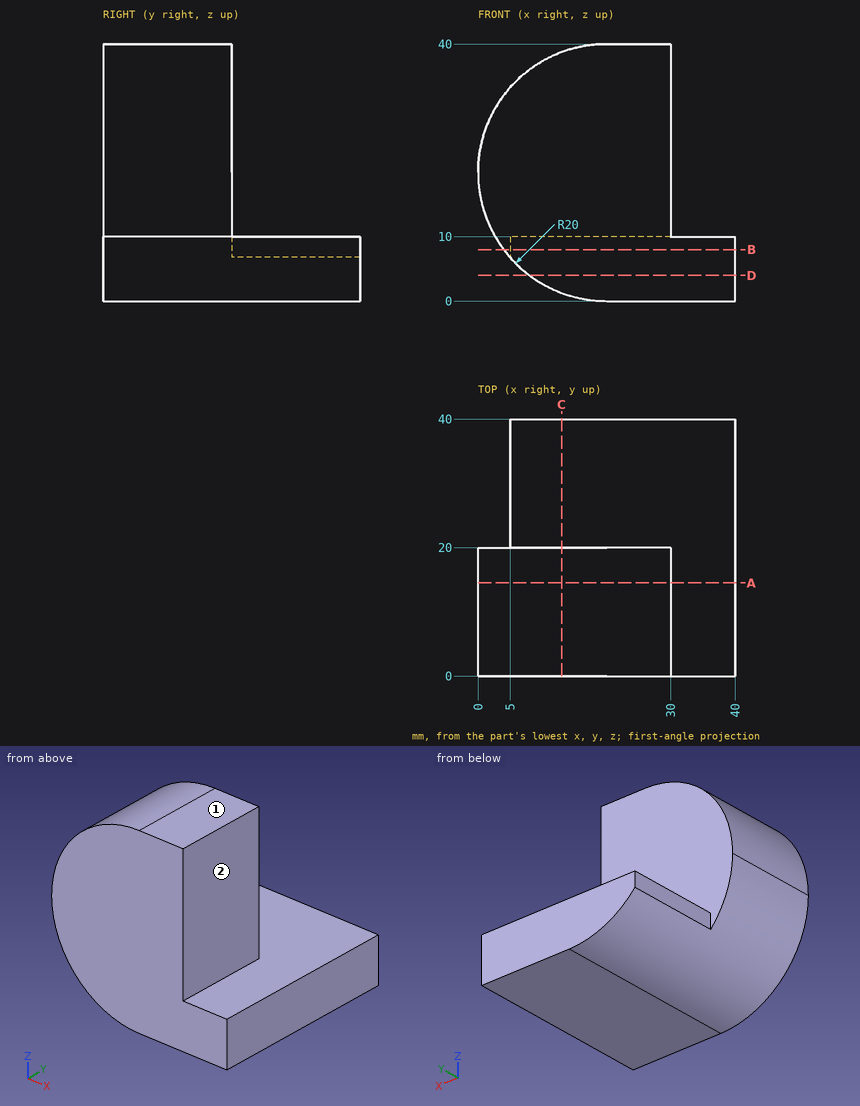
Can you work these out from the drawing? Everything is in mm from the part's minimum corner. A direction names the side the tool comes from. Round coordinates to 2 decimals unless told otherwise and drop trailing zeros. Loops run counter-clockwise (first coordinate to the right, second up) from the corner with the lowest first, then second, coordinate; pieces in that order, holes last. Notation, with made-up numbers: M 10,0 L 33,0 A33 cw 33,37 Z; hole C 71.5,45.5 d9. An arc over 180 degrees is marked long. Answer in a Markdown table with one row per item.
1. If we section it at B-B, the plane z = 8: Please give me the cut outline in (x, y).
Established:
| item | result |
|---|---|
| outline | M 4,0 L 40,0 L 40,40 L 5,40 L 5,20 L 4,20 Z |
2. On a 3-axis mill with a long thin cutter (end or side, diameter ignored), from which of +Z, -Z, +X, -X, +Y, -Y can I reach the whole of each face in a straight line? I mean the marked faces 1 and 2. Say none if no direction works.
Established:
| item | result |
|---|---|
| face 1 | +Z, +X, -X, +Y, -Y |
| face 2 | +Z, +X, +Y, -Y |
3. If we section it at D-D, the plane z = 4: Please give me the cut outline in (x, y), plus the area to 3 significant figures.
Established:
| item | result |
|---|---|
| outline | M 8,0 L 40,0 L 40,40 L 8,40 Z |
| area | 1,280 mm² |
4. If we section it at C-C, the plane x = 13: Please give me the cut outline in (y, z) (3 decimals), plus the area to 3 significant figures.
Established:
| item | result |
|---|---|
| outline | M 0,1.265 L 40,1.265 L 40,10 L 20,10 L 20,38.735 L 0,38.735 Z |
| area | 924 mm² |
5. If we section it at A-A, the plane y = 14.5: Please give me the cut outline in (x, z).
Established:
| item | result |
|---|---|
| outline | M 20,0 L 40,0 L 40,10 L 30,10 L 30,40 L 20,40 A20 ccw Z |
6. Please list where these lines run through material, in increasing order: line 1 (Y direction, x = 7.5, z = 21); line 2 (Z direction, x = 36.5, y = 11.5); line 3 (X direction, y = 15, z = 16). Write a range as from..to.
Established:
| item | result |
|---|---|
| line 1 | 0..20 |
| line 2 | 0..10 |
| line 3 | 0.4..30 |
7. I'm going to push flat-ended pins straight in: pin 1 Ø6 at (y, z) = (14, 27.5) entering from +X; pin 2 Ø1 at (x, z) = (19.5, 34) entering from +Y; pin 3 Ø2.5 at (y, z) = (31, 9) entering from -X. Where does each tip first touch, or does it pass through?
Established:
| item | result |
|---|---|
| pin 1 | x = 30 |
| pin 2 | y = 20 |
| pin 3 | x = 5 |
